CAD build for the part. Positions are in the model's coordinates, mm. A direction names the side the tool comes from. Round coordinates to 2 decimals unless told otherwise and drop trailing zeros. Loops run counter-clockwise (first coordinate to the right, second up) from the corner with the lowest first, then second, coordinate; pieces in that order, holes last.
from build123d import *

# Parameters (mm, degrees)
SKETCH1_W                 = 75
SKETCH1_H                 = 40
SKETCH1_R                 = 5
SKETCH1_R_2               = 1.7
SKETCH1_W_2               = 10
SKETCH1_H_2               = 20
BOSS_EXTRUDE1_DEPTH       = 3
CUT_EXTRUDE1_DEPTH        = 43.605750786
CUT_EXTRUDE1_DEPTH_BACK   = 43.605750786
SKETCH2_W                 = 67
SKETCH2_H                 = 28
BOSS_EXTRUDE3_DEPTH       = 110
BOSS_EXTRUDE3_DEPTH_BACK  = 3
SKETCH6_W                 = 67
SKETCH6_H                 = 11
CUT_EXTRUDE4_DEPTH        = 122.372360939
SKETCH7_W                 = 70
SKETCH7_H                 = 37
BOSS_EXTRUDE4_DEPTH       = 45
SKETCH8_W                 = 45
SKETCH8_H                 = 62
CUT_EXTRUDE6_DEPTH        = 29
SKETCH11_W                = 45
SKETCH11_H                = 4
CUT_EXTRUDE9_DEPTH        = 157.445677473
SKETCH9_W                 = 38
SKETCH9_H                 = 28.5
CUT_EXTRUDE10_DEPTH       = 204.024629048
SKETCH13_W                = 5
SKETCH13_H                = 38
BOSS_EXTRUDE5_DEPTH       = 32
SKETCH14_R                = 5
SKETCH14_R_2              = 1.7
CUT_EXTRUDE11_DEPTH       = 32
SKETCH15_W                = 165
SKETCH15_H                = 70
SKETCH15_W_2              = 157
SKETCH15_H_2              = 62
BOSS_EXTRUDE6_DEPTH       = 3
SKETCH16_W                = 20
SKETCH16_H                = 4.820648258
CUT_EXTRUDE12_DEPTH       = 159.626132778
SKETCH18_R                = 5
CUT_EXTRUDE14_DEPTH       = 159.626132778
MIRROR6_COPY_1_SKETCH_W   = 5
MIRROR6_COPY_1_SKETCH_H   = 38
MIRROR6_COPY_1_DEPTH      = 32
MIRROR6_COPY_2_SKETCH_R   = 5
MIRROR6_COPY_2_SKETCH_R_2 = 1.7
MIRROR6_COPY_2_DEPTH      = 32
SKETCH19_W                = 38
SKETCH19_H                = 3.5
CUT_EXTRUDE15_DEPTH       = 10
SKETCH20_R                = 1.2
CUT_EXTRUDE16_DEPTH       = 10
SKETCH21_W                = 10
SKETCH21_H                = 80
CUT_EXTRUDE17_DEPTH       = 184.330984833
SKETCH22_W                = 55
SKETCH22_H                = 80
CUT_EXTRUDE18_DEPTH       = 184.330984833
SKETCH23_W                = 67
SKETCH23_H                = 62
BOSS_EXTRUDE7_DEPTH       = 3
SKETCH24_R                = 10
SKETCH24_R_2              = 2.75
CUT_EXTRUDE19_DEPTH       = 111.707949127
CUT_EXTRUDE21_START       = -16
SKETCH25_R                = 5
CUT_EXTRUDE21_DEPTH       = 16


with BuildPart() as part:
    # Sketch1 → Boss-Extrude1 (new body)
    with BuildSketch(Plane(origin=(0, 0, 0), x_dir=(1, 0, 0), z_dir=(0, 1, 0))):
        Rectangle(SKETCH1_W, SKETCH1_H)
        with Locations(Location((-21, 0, 0), (0, 0, 270))):
            Circle(SKETCH1_R, mode=Mode.SUBTRACT)
        with Locations(Location((-30, 8.25, 0), (0, 0, 270))):
            Circle(SKETCH1_R_2, mode=Mode.SUBTRACT)
        with Locations(Location((-12, 8.25, 0), (0, 0, 270))):
            Circle(SKETCH1_R_2, mode=Mode.SUBTRACT)
        with Locations(Location((-12, -8.25, 0), (0, 0, 270))):
            Circle(SKETCH1_R_2, mode=Mode.SUBTRACT)
        with Locations(Location((-30, -8.25, 0), (0, 0, 270))):
            Circle(SKETCH1_R_2, mode=Mode.SUBTRACT)
        with Locations(Location((12, 8.25, 0), (0, 0, 90))):
            Circle(SKETCH1_R_2, mode=Mode.SUBTRACT)
        with Locations(Location((12, -8.25, 0), (0, 0, 90))):
            Circle(SKETCH1_R_2, mode=Mode.SUBTRACT)
        with Locations(Location((21, 0, 0), (0, 0, 90))):
            Circle(SKETCH1_R, mode=Mode.SUBTRACT)
        with Locations(Location((30, -8.25, 0), (0, 0, 90))):
            Circle(SKETCH1_R_2, mode=Mode.SUBTRACT)
        with Locations(Location((30, 8.25, 0), (0, 0, 90))):
            Circle(SKETCH1_R_2, mode=Mode.SUBTRACT)
        Rectangle(SKETCH1_W_2, SKETCH1_H_2, mode=Mode.SUBTRACT)
    extrude(amount=BOSS_EXTRUDE1_DEPTH)

    # Sketch2 → Cut-Extrude1 (cut, two sides: drawn at the far end of the back side and taken through both)
    with BuildSketch(Plane(origin=(0, 3, 0), x_dir=(1, 0, 0), z_dir=(0, 1, 0)).offset(-CUT_EXTRUDE1_DEPTH_BACK)):
        Rectangle(SKETCH2_W, SKETCH2_H)
    extrude(amount=CUT_EXTRUDE1_DEPTH + CUT_EXTRUDE1_DEPTH_BACK, mode=Mode.SUBTRACT)

    # Sketch3 → Boss-Extrude3 (add, two sides: drawn at the far end of the back side and taken through both)
    with BuildSketch(Plane(origin=(0, 3, 0), x_dir=(1, 0, 0), z_dir=(0, 1, 0)).offset(-BOSS_EXTRUDE3_DEPTH_BACK)):
        Polygon((37.5, -35), (37.5, -20), (33.5, -20), (-33.5, -20), (-37.5, -20), (-37.5, -35), align=None)
        Polygon((33.5, 20), (37.5, 20), (37.5, 35), (-37.5, 35), (-37.5, 20), (-33.5, 20), align=None)
        Polygon((37.5, -20), (37.5, 20), (33.5, 20), (33.5, 14), (33.5, -14), (33.5, -20), align=None)
        Polygon((-33.5, 14), (-33.5, 20), (-37.5, 20), (-37.5, -20), (-33.5, -20), (-33.5, -14), align=None)
    extrude(amount=BOSS_EXTRUDE3_DEPTH + BOSS_EXTRUDE3_DEPTH_BACK)

    # Sketch6 → Cut-Extrude4 (cut, through all)
    with BuildSketch(Plane(origin=(0, 3, 0), x_dir=(1, 0, 0), z_dir=(0, 1, 0))):
        with Locations((0, -25.5)):
            Rectangle(SKETCH6_W, SKETCH6_H)
        with Locations((0, 25.5)):
            Rectangle(SKETCH6_W, SKETCH6_H)
    extrude(amount=CUT_EXTRUDE4_DEPTH, mode=Mode.SUBTRACT)

    # Sketch7 → Boss-Extrude4 (add)
    with BuildSketch(Plane.ZY.offset(37.5)):
        with Locations((0, 94.5)):
            Rectangle(SKETCH7_W, SKETCH7_H)
    boss_extrude4 = extrude(amount=BOSS_EXTRUDE4_DEPTH)

    # Mirror2: Boss-Extrude4 across plane
    add(boss_extrude4.mirror(Plane(origin=(0, 0, 0), x_dir=(0, 0, 1), z_dir=(1, 0, 0))))

    # Sketch8 → Cut-Extrude6 (cut)
    with BuildSketch(Plane(origin=(0, 113, 0), x_dir=(1, 0, 0), z_dir=(0, 1, 0))):
        with Locations((-56, 0)):
            Rectangle(SKETCH8_W, SKETCH8_H)
        with Locations((56, 0)):
            Rectangle(SKETCH8_W, SKETCH8_H)
    extrude(amount=-CUT_EXTRUDE6_DEPTH, mode=Mode.SUBTRACT)

    # Sketch11 → Cut-Extrude9 (cut, through all)
    with BuildSketch(Plane.XY.offset(35)):
        with Locations((-60, 78)):
            Rectangle(SKETCH11_W, SKETCH11_H)
        with Locations((60, 78)):
            Rectangle(SKETCH11_W, SKETCH11_H)
    extrude(amount=-CUT_EXTRUDE9_DEPTH, mode=Mode.SUBTRACT)

    # Sketch9 → Cut-Extrude10 (cut, through all)
    with BuildSketch(Plane.ZY.offset(82.5)):
        with Locations((0, 98.25)):
            Rectangle(SKETCH9_W, SKETCH9_H)
    extrude(amount=-CUT_EXTRUDE10_DEPTH, mode=Mode.SUBTRACT)

    # Sketch13 → Boss-Extrude5 (add)
    with BuildSketch(Plane(origin=(0, 84, 0), x_dir=(1, 0, 0), z_dir=(0, 1, 0))):
        with Locations((-54.5, 0)):
            Rectangle(SKETCH13_W, SKETCH13_H)
    boss_extrude5 = extrude(amount=BOSS_EXTRUDE5_DEPTH)

    # Sketch14 → Cut-Extrude11 (cut)
    with BuildSketch(Plane.ZY.offset(57)):
        with Locations((0, 101)):
            Circle(SKETCH14_R)
        with Locations((-8.25, 110)):
            Circle(SKETCH14_R_2)
        with Locations((8.25, 110)):
            Circle(SKETCH14_R_2)
        with Locations((8.25, 92)):
            Circle(SKETCH14_R_2)
        with Locations((-8.25, 92)):
            Circle(SKETCH14_R_2)
    cut_extrude11 = extrude(amount=-CUT_EXTRUDE11_DEPTH, mode=Mode.SUBTRACT)

    # Mirror4: Boss-Extrude5, Cut-Extrude11 across plane
    add(boss_extrude5.mirror(Plane(origin=(0, 0, 0), x_dir=(0, 0, 1), z_dir=(1, 0, 0))))
    add(cut_extrude11.mirror(Plane(origin=(0, 0, 0), x_dir=(0, 0, 1), z_dir=(1, 0, 0))), mode=Mode.SUBTRACT)

    # Sketch15 → Boss-Extrude6 (add)
    with BuildSketch(Plane(origin=(0, 113, 0), x_dir=(1, 0, 0), z_dir=(0, 1, 0))):
        Rectangle(SKETCH15_W, SKETCH15_H)
        Rectangle(SKETCH15_W_2, SKETCH15_H_2, mode=Mode.SUBTRACT)
    extrude(amount=BOSS_EXTRUDE6_DEPTH)

    # Sketch16 → Cut-Extrude12 (cut, through all)
    with BuildSketch(Plane.XY.offset(35)):
        with Locations((0, 11.636111214)):
            Rectangle(SKETCH16_W, SKETCH16_H)
    extrude(amount=-CUT_EXTRUDE12_DEPTH, mode=Mode.SUBTRACT)

    # Sketch18 → Cut-Extrude14 (cut, through all)
    with BuildSketch(Plane.XY.offset(35)):
        with Locations((67.75, 100)):
            Circle(SKETCH18_R)
    cut_extrude14 = extrude(amount=-CUT_EXTRUDE14_DEPTH, mode=Mode.SUBTRACT)

    # Mirror5: Cut-Extrude14 across plane
    add(cut_extrude14.mirror(Plane(origin=(0, 0, 0), x_dir=(0, 0, 1), z_dir=(1, 0, 0))), mode=Mode.SUBTRACT)

    # Mirror6: Boss-Extrude5, Cut-Extrude11 across plane
    add(boss_extrude5.mirror(Plane.ZX.offset(116)))
    add(cut_extrude11.mirror(Plane.ZX.offset(116)), mode=Mode.SUBTRACT)

    # Mirror6 copy 1 sketch → Mirror6 copy 1 (add)
    with BuildSketch(Plane(origin=(0, 148, 0), x_dir=(-1, 0, 0), z_dir=(0, -1, 0))):
        with Locations((-54.5, 0)):
            Rectangle(MIRROR6_COPY_1_SKETCH_W, MIRROR6_COPY_1_SKETCH_H)
    extrude(amount=MIRROR6_COPY_1_DEPTH)

    # Mirror6 copy 2 sketch → Mirror6 copy 2 (cut)
    with BuildSketch(Plane(origin=(57, 232, 0), x_dir=(0, 0, 1), z_dir=(1, 0, 0))):
        with Locations((0, 101)):
            Circle(MIRROR6_COPY_2_SKETCH_R)
        with Locations((-8.25, 110)):
            Circle(MIRROR6_COPY_2_SKETCH_R_2)
        with Locations((8.25, 110)):
            Circle(MIRROR6_COPY_2_SKETCH_R_2)
        with Locations((8.25, 92)):
            Circle(MIRROR6_COPY_2_SKETCH_R_2)
        with Locations((-8.25, 92)):
            Circle(MIRROR6_COPY_2_SKETCH_R_2)
    extrude(amount=-MIRROR6_COPY_2_DEPTH, mode=Mode.SUBTRACT)

    # Sketch19 → Cut-Extrude15 (cut)
    with BuildSketch(Plane(origin=(82.5, 0, 0), x_dir=(0, 0, -1), z_dir=(1, 0, 0))):
        with Locations((0, 114.25)):
            Rectangle(SKETCH19_W, SKETCH19_H)
    cut_extrude15 = extrude(amount=-CUT_EXTRUDE15_DEPTH, mode=Mode.SUBTRACT)

    # Mirror7: Cut-Extrude15 across plane
    add(cut_extrude15.mirror(Plane(origin=(0, 0, 0), x_dir=(0, 0, 1), z_dir=(1, 0, 0))), mode=Mode.SUBTRACT)

    # Sketch20 → Cut-Extrude16 (cut)
    with BuildSketch(Plane(origin=(0, 3, 0), x_dir=(1, 0, 0), z_dir=(0, 1, 0))):
        with Locations(Location((-24, 17.5, 0), (0, 0, 270))):
            Circle(SKETCH20_R)
        with Locations(Location((-12, 17.5, 0), (0, 0, 270))):
            Circle(SKETCH20_R)
        with Locations(Location((12, 17.5, 0), (0, 0, 270))):
            Circle(SKETCH20_R)
        with Locations(Location((-24, -17.5, 0), (0, 0, 270))):
            Circle(SKETCH20_R)
        with Locations(Location((-12, -17.5, 0), (0, 0, 270))):
            Circle(SKETCH20_R)
        with Locations(Location((24, 17.5, 0), (0, 0, 270))):
            Circle(SKETCH20_R)
        with Locations(Location((12, -17.5, 0), (0, 0, 270))):
            Circle(SKETCH20_R)
        with Locations(Location((24, -17.5, 0), (0, 0, 270))):
            Circle(SKETCH20_R)
    extrude(amount=-CUT_EXTRUDE16_DEPTH, mode=Mode.SUBTRACT)

    # Sketch21 → Cut-Extrude17 (cut, through all)
    with BuildSketch(Plane.XY.offset(35)):
        with Locations((32.5, 40)):
            Rectangle(SKETCH21_W, SKETCH21_H)
        with Locations((-32.5, 40)):
            Rectangle(SKETCH21_W, SKETCH21_H)
    extrude(amount=-CUT_EXTRUDE17_DEPTH, mode=Mode.SUBTRACT)

    # Sketch22 → Cut-Extrude18 (cut, through all)
    with BuildSketch(Plane.XY.offset(35)):
        with Locations((0, 40)):
            Rectangle(SKETCH22_W, SKETCH22_H)
    extrude(amount=-CUT_EXTRUDE18_DEPTH, mode=Mode.SUBTRACT)

    # Sketch23 → Boss-Extrude7 (add)
    with BuildSketch(Plane.XZ.offset(-80)):
        Rectangle(SKETCH23_W, SKETCH23_H)
    extrude(amount=-BOSS_EXTRUDE7_DEPTH)

    # Sketch24 → Cut-Extrude19 (cut, through all)
    with BuildSketch(Plane(origin=(0, 83, 0), x_dir=(1, 0, 0), z_dir=(0, 1, 0))):
        with Locations(Location((0, 0, 0), (0, 0, 270))):
            Circle(SKETCH24_R)
        with Locations(Location((-20, 19, 0), (0, 0, 270))):
            Circle(SKETCH24_R_2)
        with Locations(Location((-20, -19, 0), (0, 0, 270))):
            Circle(SKETCH24_R_2)
        with Locations(Location((20, -19, 0), (0, 0, 90))):
            Circle(SKETCH24_R_2)
        with Locations(Location((20, 19, 0), (0, 0, 90))):
            Circle(SKETCH24_R_2)
    extrude(amount=-CUT_EXTRUDE19_DEPTH, mode=Mode.SUBTRACT)

    # Sketch25 → Cut-Extrude21 (cut)
    with BuildSketch(Plane(origin=(0, 0, -35), x_dir=(-1, 0, 0), z_dir=(0, 0, -1)).offset(CUT_EXTRUDE21_START)):
        Polygon((33.5, 116), (33.5, 84), (33.5, 80), (82.5, 80), (82.5, 116), align=None)
        with Locations((67.75, 100)):
            Circle(SKETCH25_R, mode=Mode.SUBTRACT)
    cut_extrude21 = extrude(amount=CUT_EXTRUDE21_DEPTH, mode=Mode.SUBTRACT)

    # Mirror8: Cut-Extrude21 across plane
    add(cut_extrude21.mirror(Plane(origin=(0, 0, 0), x_dir=(0, 0, 1), z_dir=(1, 0, 0))), mode=Mode.SUBTRACT)


solid = part.part
Item 1: 3-axis set-ups, long thin cutter, end or side, ignore diameter. For faces 1 (the cylindrical face through (-54.54, 90.34, 7.88)), 2 (the flat face through (52, 116, 0)), 3 (the flat face through (-56, 104, -19)), 4 (the flat face through (-55, 116, 19)): which of +Z, -Z, +X, -X, +Y, -Y reach the whole face in a straight line?
Verdict:
face 1: +X, -X
face 2: -Z, +Y
face 3: -Z, -X, +Y, -Y
face 4: +Y
Item 2: Cut at C-C (z = 24). List the corners of the cut face in (x, y), plus the area to 3 significant figures.
Verdict:
outline: (-82.5, 80) - (82.5, 80) - (82.5, 116) - (78.5, 116) - (78.5, 84) - (33.5, 84) - (33.5, 83) - (-33.5, 83) - (-33.5, 84) - (-78.5, 84) - (-78.5, 116) - (-82.5, 116) - close
area: 849 mm2
Item 3: Wall check: L1, parallel to Y at x = 53.9, z = -8.25; L2, parallel to Z at x = -54, y = 140; L3, parallel to Z at x = 13.5, y = 110. Give the ranges that are in metal, low to high.
Verdict:
L1: y = 80 to 90.3, 93.7 to 108.3, 111.7 to 120.3, 123.7 to 138.3, 141.7 to 148
L2: z = -19 to -9.95, -6.55 to 6.55, 9.95 to 19
L3: z = -35 to -31, 31 to 35
Item 4: Cut at B-B (x = -20). List the corners of the cut face in (y, z).
Verdict:
outline: (80, -35) - (116, -35) - (116, -31) - (83, -31) - (83, -21.75) - (80, -21.75) - close; (80, -16.25) - (83, -16.25) - (83, 16.25) - (80, 16.25) - close; (80, 21.75) - (83, 21.75) - (83, 31) - (116, 31) - (116, 35) - (80, 35) - close
Item 5: Cut at D-D (y = 110). State how many separate pieces and enclosed holes the cut face has, plus the area to 3 significant figures.
Verdict:
separate pieces: 8
enclosed holes: 0
area: 1,340 mm2
Item 6: Mould opens along X. For faces 5 (the flat face through (57, 116, 0)), 6 (the flat face through (-8, 83, 7)), 7 (the cylindrical face through (-54.54, 108.34, 7.88)) say: released by +X, released by -X, zero draft, split by the parting line, or undercut.
Verdict:
face 5: released by +X
face 6: undercut
face 7: zero draft
Item 7: Flat gauge pins, fed straight in: P1, Ø1, axis at x = 46.5, z = 21, coming from the +Y side; P2, Ø3, axis at y = 103.5, z = -6.5, coming from the +X side; P3, Ø4.5, axis at y = 122, z = 8.25, coming from the -X side; P4, Ø12, axis at x = 0, z = 0, coming from the +Y side. Where does each tip first touch, or does it go through?
Verdict:
P1: stops at y = 84
P2: stops at x = 57
P3: stops at x = -57
P4: passes through
Item 8: Cut at A-A (x = -67.75). List the corners of the cut face in (y, z).
Verdict:
outline: (80, -19) - (84, -19) - (84, 31) - (95, 31) - (95, 35) - (80, 35) - close; (105, 31) - (116, 31) - (116, 35) - (105, 35) - close
